Can you work these out from the model? Positions are in its coordinate system, mm. A direction names the side the tool comes from. Give positions to 0.01 mm unless a question says otherwise; leave off trailing zeros. Loops run counter-clockwise (first coordinate to the right, second up) from the corner with the lowest first, then second, coordinate; pieces in that order, holes last. Notation, with made-up numbers: (37, 77.25) - (60, 77.25) arc R32 ccw to (60, 106.25) - close; hole circle Ø5 at (15.5, 88.25). An arc over 180 degrees is marked (long way). Answer as a JSON object with one key per item and string values. Group by question number.
Item 1: Thinking about a two-plate mould opening in Y: for faces 1 (the flat face through (-7, -48, 0)), 2 (the cylindrical face through (-6.38, -48.54, 0.89)), 3 (the flat face through (0, -37, 1)), which applies, pulls with the +Y half, pulls with the -Y half, needs draft (parallel to the pull), parting line crosses it, or undercut?
Item 2: Suppose I cut it at C-C on x = -11.25. Write out the boundary of the cut face in (y, z), and give its area (3 significant figures).
Item 3: Suppose I cut it at B-B on y = -50.25. Write out the boundary of the cut face in (x, z).
Item 4: Will these pins go through, and if not, where does the flat tip stop? pin 1 (1 mm diameter, centred on y = -50.5, z = 3, fed in from +X); pin 2 (3.5 mm diameter, centred on x = -5, y = -44.5, fed in from -Z); pin 3 (0.7 mm diameter, centred on y = -44, z = 0.5, fed in from -X).
Item 5: Please list where these lines run through material, in increasing order: L1, parallel to Y at x = 6, z = 1.2; L2, parallel to X at y = -49.5, z = 0.5; L3, parallel to X at y = -46, z = 3.
Item 6: Which directions (+Z, -Z, +X, -X, +Y, -Y) give clear straight access to the entire face, cutting with the end or side of a thin tool? Please do faces 4 (the flat face through (-8.5, -40, 0)), 5 (the flat face through (3.25, -46, 1)), 6 (the flat face through (8.5, -40, 0)).
Item 7: Suppose I cut it at A-A on z = -1.25. Write out the boundary of the cut face in (x, y), and give its area (3 significant figures).
Autodesk Inventor part; units mm, degrees
ref_plane "Płaszczyzna konstrukcyjna1" through (0, 0, 0) normal (0, 0, 1) x (1, 0, 0)
ref_plane "Płaszczyzna konstrukcyjna2" through (0, -53, 0) normal (1, 0, 0) x (0, 0, -1)
ref_plane "YZ Plane" through (0, 0, 0) normal (1, 0, 0) x (0, 1, 0)
ref_plane "Płaszczyzna konstrukcyjna1" through (0, 0, 0) normal (0, 0, 1) x (1, 0, 0)
sketch "Szkic1" plane through (0, 0, 0) normal (0, 0, 1) x (1, 0, 0)
  circle A0 centre (6, -50.25) radius 1.75
  circle A1 centre (-6, -50.25) radius 1.75
  circle A2 centre (6, -3.75) radius 1.75 construction
  circle A3 centre (-6, -3.75) radius 1.75 construction
  arc A4 (7, -56) -> (10, -53) centre (7, -53) ccw
  line L0 (10, -53) -> (10, -45)
  arc A5 (10, -45) -> (7, -42) centre (7, -45) ccw
  line L1 (7, -42) -> (5, -42)
  line L2 (5, -42) -> (5, -12) construction
  line L3 (5, -12) -> (7, -12) construction
  arc A6 (7, -12) -> (10, -9) centre (7, -9) ccw construction
  line L4 (10, -9) -> (10, -1) construction
  arc A7 (10, -1) -> (7, 2) centre (7, -1) ccw construction
  line L5 (7, 2) -> (-7, 2) construction
  arc A8 (-7, 2) -> (-10, -1) centre (-7, -1) ccw construction
  line L6 (-10, -1) -> (-10, -9) construction
  arc A9 (-10, -9) -> (-7, -12) centre (-7, -9) ccw construction
  line L7 (-7, -12) -> (-5, -12) construction
  line L8 (-5, -12) -> (-5, -42) construction
  line L9 (-5, -42) -> (-7, -42)
  arc A10 (-7, -42) -> (-10, -45) centre (-7, -45) ccw
  line L10 (-10, -45) -> (-10, -53)
  arc A11 (-10, -53) -> (-7, -56) centre (-7, -53) ccw
  line L11 (-7, -56) -> (7, -56)
  line L12 (-5.5, -42) -> (5.5, -42)
  line L13 (5.5, -42) -> (5.5, -37)
  line L14 (5.5, -37) -> (-5.5, -37)
  line L15 (-5.5, -37) -> (-5.5, -42)
  line L16 (0, -56) -> (0, 2) construction
  line L17 (-5.5, -37) -> (-8.5, -37)
  line L18 (-8.5, -37) -> (-8.5, -42)
  line L19 (-8.5, -42) -> (-5.5, -42)
  line L20 (-5.5, -42) -> (-5.5, -37)
  line L21 (5.5, -37) -> (8.5, -37)
  line L22 (8.5, -37) -> (8.5, -42)
  line L23 (8.5, -42) -> (5.5, -42)
  line L24 (5.5, -42) -> (5.5, -37)
  line L25 (-8.5, -42) -> (-8.5, -42.4019)
  line L26 (8.5, -42) -> (8.5, -42.4019)
  dimension "d0" = 11
  dimension "d1" = 3
  dimension "d2" = 3
  dimension "d3" = 5
extrude "Wyciągnięcie proste1" add sketch "Szkic1" along normal blind 4
ref_plane "Płaszczyzna konstrukcyjna2" through (0, -53, 0) normal (1, 0, 0) x (0, 0, -1)
sketch "Szkic2" plane through (0, -53, 0) normal (1, 0, 0) x (0, 0, -1)
  line L0 (0, -3) -> (-4, -3)
  line L1 (-4, -3) -> (-4, 16)
  line L2 (-4, 16) -> (0, 16)
  line L3 (0, 16) -> (0, -3)
  line L4 (-1.4, -3) -> (-1.4, -1) construction
  line L5 (-1.4, -3) -> (-1.4, -2.4)
  line L6 (-1.4, -2.4) -> (-1.2, -2.4)
  arc A0 (-1.2, -2.4) -> (-1.2, -1.6) centre (-1.2, -2) ccw
  line L7 (-1.2, -1.6) -> (-1.4, -1.6)
  line L8 (-1.4, -1.6) -> (-1.4, -1)
  line L9 (-1.4, -2) -> (-1.2, -2) construction
  line L10 (-1.4, -1) -> (0, -1)
  line L11 (0, -1) -> (0, -3)
  line L12 (0, -3) -> (-1.4, -3)
  point P0 (0, 53)
  dimension "d6" = 2
  dimension "d7" = 1.4
  dimension "d8" = 0.4
  dimension "d9" = 0.2
extrude "Wyciągnięcie proste2" cut sketch "Szkic2" along normal mid plane 6.5 contours L0 L5 L6 A0 L7 L8 L10 L3
pattern_linear "Szyk prostokątny1" count 10 spacing 2 along (0, 1, 0) of "Wyciągnięcie proste2"
sketch "Szkic3" plane through (0, 0, 4) normal (0, 0, 1) x (1, 0, 0)
  circle A0 centre (-6, -50.25) radius 1.75
  circle A1 centre (6, -50.25) radius 1.75
  line L0 (10, -53) -> (10, -45)
  line L1 (-6, -46.7859) -> (-3, -48.5179)
  line L2 (-3, -48.5179) -> (-3, -51.9821)
  line L3 (-3, -51.9821) -> (-6, -53.7141)
  line L4 (-6, -53.7141) -> (-9, -51.9821)
  line L5 (-9, -51.9821) -> (-9, -48.5179)
  line L6 (-9, -48.5179) -> (-6, -46.7859)
  line L7 (6, -46.7859) -> (9, -48.5179)
  line L8 (9, -48.5179) -> (9, -51.9821)
  line L9 (9, -51.9821) -> (6, -53.7141)
  line L10 (6, -53.7141) -> (3, -51.9821)
  line L11 (3, -51.9821) -> (3, -48.5179)
  line L12 (3, -48.5179) -> (6, -46.7859)
  point P0 (0, 0)
  dimension "d23" = 6
  dimension "d24" = 6
extrude "Wyciągnięcie proste3" cut sketch "Szkic3" against normal blind 2
sketch "Szkic4" plane through (0, 0, 0) normal (0, 0, -1) x (-1, 0, 0)
  line L0 (8.5, -37) -> (8.5, -42.4019)
  line L1 (3.25, -37) -> (8.5, -37)
  line L2 (-5.5, -42) -> (-5.5, -37)
  line L3 (-8.5, -42) -> (-5.5, -42)
  line L4 (5.5, -42) -> (5.5, -37)
  line L5 (8.5, -42) -> (5.5, -42)
  line L6 (-3.25, -56) -> (-3.25, -37)
  line L7 (-8.5, -37) -> (-3.25, -37)
  line L8 (-8.5, -42.4019) -> (-8.5, -37)
  arc A0 (-8.5, -42.4019) -> (-10, -45) centre (-7, -45) ccw
  line L9 (-10, -53) -> (-10, -45)
  arc A1 (-10, -53) -> (-7, -56) centre (-7, -53) ccw
  line L10 (-3.25, -56) -> (-7, -56)
  circle A2 centre (-6, -50.25) radius 1.75
  line L11 (-8.5, -42) -> (-8.5, -37)
  line L12 (-8.5, -37) -> (-5.5, -37)
  point P0 (0, 0)
extrude "Wyciągnięcie proste4" add sketch "Szkic4" along normal blind 3 contours L0 L5 L4 L1 | L3 L8 L7 L2
sketch "Szkic5" plane through (6, -50.25, 2) normal (0, 0, 1) x (1, 0, 0)
  circle A0 centre (0, 0) radius 1.75
  circle A1 centre (-12, 0) radius 1.75
  point P0 (-6, 50.25)
extrude "Wyciągnięcie proste5" add sketch "Szkic5" against normal blind 0.2
sketch "Szkic6" plane through (0, 0, 4) normal (0, 0, 1) x (1, 0, 0)
  line L0 (8.5, -37) -> (-8.5, -37)
  line L1 (-8.5, -37) -> (-8.5, -42.4019)
  arc A0 (-8.5, -42.4019) -> (-10, -45) centre (-7, -45) ccw
  line L2 (-10, -45) -> (-10, -53)
  arc A1 (-10, -53) -> (-7, -56) centre (-7, -53) ccw
  line L3 (-7, -56) -> (7, -56)
  arc A2 (7, -56) -> (10, -53) centre (7, -53) ccw
  line L4 (10, -53) -> (10, -45)
  arc A3 (10, -45) -> (8.5, -42.4019) centre (7, -45) ccw
  line L5 (8.5, -42.4019) -> (8.5, -37)
  line L6 (-11.6786, -33.8214) -> (11.6786, -33.8214)
  line L7 (11.6786, -33.8214) -> (11.6786, -40.9644)
  arc A4 (13.1786, -45) -> (11.6786, -40.9644) centre (7, -45) ccw
  line L8 (13.1786, -45) -> (13.1786, -53)
  arc A5 (7, -59.1786) -> (13.1786, -53) centre (7, -53) ccw
  line L9 (7, -59.1786) -> (-7, -59.1786)
  arc A6 (-13.1786, -53) -> (-7, -59.1786) centre (-7, -53) ccw
  line L10 (-13.1786, -53) -> (-13.1786, -45)
  arc A7 (-11.6786, -40.9644) -> (-13.1786, -45) centre (-7, -45) ccw
  line L11 (-11.6786, -40.9644) -> (-11.6786, -33.8214)
  point P0 (0, 0)
extrude "Wyciągnięcie proste6" add sketch "Szkic6" against normal blind 0.2
properties part number "bed_belt_clip"
Worked out:
{
 "1": {"face 1": "needs draft", "face 2": "undercut", "face 3": "pulls with the +Y half"},
 "2": {"outline": "(-57.48, 3.8) - (-33.82, 3.8) - (-33.82, 4) - (-57.48, 4) - close", "area": "4.73 mm2"},
 "3": {"outline": "(-13.18, 3.8) - (-10, 3.8) - (-10, 0) - (-7.75, 0) - (-7.75, 1.8) - (-4.25, 1.8) - (-4.25, 0) - (-3.25, 0) - (-3.25, 1.4) - (3.25, 1.4) - (3.25, 0) - (4.25, 0) - (4.25, 1.8) - (7.75, 1.8) - (7.75, 0) - (10, 0) - (10, 3.8) - (13.18, 3.8) - (13.18, 4) - (9, 4) - (9, 2) - (3, 2) - (3, 4) - (-3, 4) - (-3, 2) - (-9, 2) - (-9, 4) - (-13.18, 4) - close"},
 "4": {"pin 1": "stops at x = 10", "pin 2": "stops at z = 0", "pin 3": "stops at x = -9.93"},
 "5": {"L1": "y = -56 to -52, -48.5 to -37", "L2": "x = -10 to -7.58, -4.42 to -3.25, 3.25 to 4.42, 7.58 to 10", "L3": "x = -10 to 10"},
 "6": {"face 4": "-Z, -X, +Y", "face 5": "-Z", "face 6": "-Z, +X, +Y"},
 "7": {"outline": "(-8.5, -42) - (-5.5, -42) - (-5.5, -37) - (-8.5, -37) - close; (5.5, -42) - (8.5, -42) - (8.5, -37) - (5.5, -37) - close", "area": "30.0 mm2"}
}
